The figure shows three views and two pictorial views of one solid part (mm, origin at its lowest corner). Answer the questions. A direction names the side the tool comes from. Give positions to 0.01 mm unless a question says otherwise; leave off trailing zeros. Order: outer loops, then holes, each group sorted by start corner. A loop starts at its lowest first (then second) coordinate and runs counter-clockwise, first axis right, second up. Notation, with made-up numbers: M -21,-14.5 L -1,-14.5 A18 ccw -1,-2.5 Z; hole C 70.25,87 d4. An arc over 180 degrees is marked long. Answer as a JSON object with one key per item and string values. Group by question number.
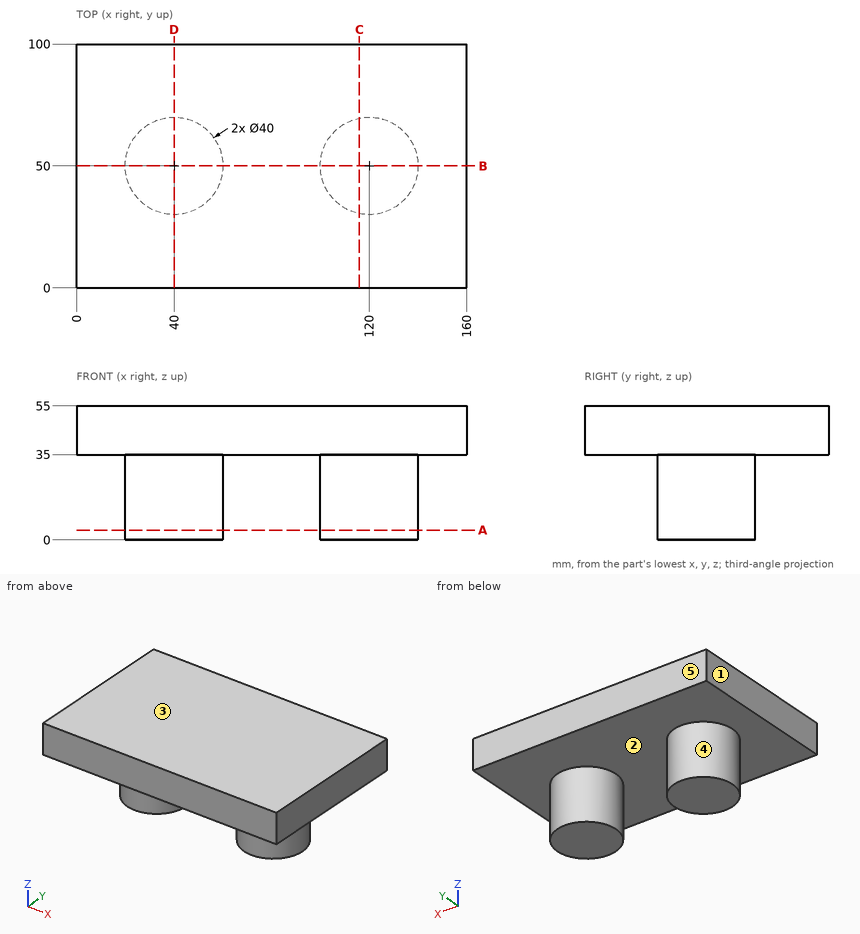
Item 1: Determine the mould class of the marked faces 1, 2 and 3 for opening direction X: released by +X, released by -X, zero draft, split by the parting line, or undercut.
Item 2: Section B-B (y = 50) is taken. Determine the outline of the cut face in (x, z), and give its area (3 significant figures).
Item 3: Section A-A (z = 4) is taken. Determine the outline of the cut face in (x, y), and give its area (3 significant figures).
Item 4: Consider probe 1 along Z at (x, y) = (50, 8); probe 2 along X at (y, z) = (39, 17); probe 3 along Y at (x, z) = (119.5, 14.5). Determine where each line is inside the solid, lowest interval first. Write a range as from..to.
Item 5: Section C-C (x = 116) is taken. Determine the outline of the cut face in (y, z), and give its area (3 significant figures).
Item 6: Flat-ended cylindrical pins translate along their axes: P1, Ø1.5, axis at x = 48.5, z = 20.5, coming from the +Y side; P2, Ø1.5, axis at x = 33.5, y = 74.5, coming from the -Z side; P3, Ø4, axis at y = 74, z = 32.5, coming from the -X side. Find the tip coordinate at first contact, or state that the pin passes through.
Item 7: A tool of negligible diameter and unlimited length cuts with its end or side. For the marked faces 4 and 5, from which of +Z, -Z, +X, -X, +Y, -Y can it reach the whole face along a straight path? Write none if from no direction.
Item 8: Section D-D (x = 40) is taken. Determine the outline of the cut face in (y, z), and give its area (3 significant figures).
Values found:
{
 "1": {"face 1": "released by -X", "face 2": "undercut", "face 3": "zero draft"},
 "2": {"outline": "M 0,35 L 20,35 L 20,0 L 60,0 L 60,35 L 100,35 L 100,0 L 140,0 L 140,35 L 160,35 L 160,55 L 0,55 Z", "area": "6,000 mm^2"},
 "3": {"outline": "C 40,50 d40; C 120,50 d40", "area": "2,510 mm^2"},
 "4": {"probe 1": "z = 35..55", "probe 2": "x = 23.3..56.7, 103.3..136.7", "probe 3": "y = 30.01..69.99"},
 "5": {"outline": "M 0,35 L 30.4,35 L 30.4,0 L 69.6,0 L 69.6,35 L 100,35 L 100,55 L 0,55 Z", "area": "3,370 mm^2"},
 "6": {"P1": "stops at y = 68.44", "P2": "stops at z = 35", "P3": "passes through"},
 "7": {"face 4": "-Z", "face 5": "+Z, -Z, +X, -X, +Y"},
 "8": {"outline": "M 0,35 L 30,35 L 30,0 L 70,0 L 70,35 L 100,35 L 100,55 L 0,55 Z", "area": "3,400 mm^2"}
}
